Input: part model. Units: mm. Frame: model coordinates. A direction names the side the tool comes from. Round coordinates to 2 decimals unless told otherwise and drop trailing zeros. Order: outer loops, then holes, each group sorted by start corner. A loop starts at its lowest first (then second) coordinate and runs counter-clockwise, first axis right, second up. Notation, with made-up numbers: (-14, -7) -> (14, -7) arc R20 ccw to (14, 0) -> close; hole circle Ø11 at (-19.5, 26). An arc over 180 degrees is marked (long way). Answer as CSV lines item,"result". Start each with the question number.
1) Line query: L1, parallel to Y at x = 0, z = 13.25; L2, parallel to Z at x = -4.5, y = 12; L3, parallel to Z at x = -8.5, y = 1.5. Output: solid intervals per line, ascending.
2) First-contact query: P1, Ø2, axis at y = -2.5, z = 11, coming from the +X side; P2, Ø1, axis at x = -12, y = 8, coming from the +Z side; P3, Ø1.5, axis at x = 1.5, z = 9.5, coming from the -Y side. Flat tips, straight axial feed; report the tip coordinate or a pass-through.
3) Mould query, pull axis Y, two halves, no side actions, for faces 3 (the face through (-2.63, -11.86, 10.38)), 4 (the face through (0, 0, 1.6)), 5 (the face through (-4, 10, 19)). Classes: +Y half, -Y half, draft (parallel to the pull), parting line (faces both ways), or undercut.
4) Section query C-C, the plane z = 5. Output: boundary loops of the cut face in (x, y).
5) Section query A-A, the plane y = 0. Output: boundary loops of the cut face in (x, z).
6) Access query for faces 1 (the face through (-13.887, -10.648, 0.986)), 2 (the face through (-12, -4, 2)). Directions: +Z, -Z, +X, -X, +Y, -Y. A direction counts if a zero-diameter tool reaches every point of the face in a straight line with its end or side. Return the directions, or none.
```python
from build123d import *

# Parameters (mm, degrees)
F0_R     = 17.5
F1_DEPTH = 2
F2_R     = 12.15
F3_DEPTH = 17
F4_T     = -1.6


with BuildPart() as f1:
    # F0 (on Top) → F1 (new body)
    with BuildSketch(Plane.XY):
        Circle(F0_R)
    extrude(amount=F1_DEPTH)

    # F2 (on face) → F3 (join)
    with BuildSketch(Plane.XY.offset(2)):
        Circle(F2_R)
    extrude(amount=F3_DEPTH)

    # F4
    f4_openings = [f1.faces().sort_by_distance(p)[0] for p in [
        (0, 0, 19),
    ]]
    offset(amount=F4_T, openings=f4_openings, kind=Kind.INTERSECTION)


solid = f1.part
```
Findings:
1,L1,"y = -12.15 to -10.55, 10.55 to 12.15"
1,L2,"z = 0 to 2"
1,L3,"z = 0 to 1.6"
2,P1,"stops at x = 12.06"
2,P2,"stops at z = 2"
2,P3,"stops at y = -12.13"
3,face 3,"parting line"
3,face 4,"undercut"
3,face 5,"draft"
4,outline,"circle Ø24.3 at (0, 0); hole circle Ø21.1 at (0, 0)"
5,outline,"(-17.5, 0) -> (17.5, 0) -> (17.5, 2) -> (12.15, 2) -> (12.15, 19) -> (10.55, 19) -> (10.55, 1.6) -> (-10.55, 1.6) -> (-10.55, 19) -> (-12.15, 19) -> (-12.15, 2) -> (-17.5, 2) -> close"
6,face 1,"+Z, -Z"
6,face 2,"+Z"
